Here's how the part is built. I have some questions about the finished solid (model axes, mm). A direction names the side the tool comes from. Coordinates: 2 decimals unless noted, no trailing zeros. Order: outer loops, then holes, each group sorted by start corner. A loop starts at its lowest first (then second) coordinate and runs counter-clockwise, first axis right, second up.
Autodesk Inventor part; units mm, degrees
ref_plane "YZ Plane" through (0, 0, 0) normal (1, 0, 0) x (0, 1, 0)
ref_plane "XZ Plane" through (0, 0, 0) normal (0, 1, 0) x (-1, 0, 0)
ref_plane "XY Plane" through (0, 0, 0) normal (0, 0, 1) x (1, 0, 0)
sketch "Sketch1" plane through (0, 0, 0) normal (0, 1, 0) x (-1, 0, 0)
  line L0 (-65.5034, 14.4772) -> (4.4966, 14.4772)
  line L1 (4.4966, 14.4772) -> (4.4966, -155.5228)
  line L2 (4.4966, -155.5228) -> (-65.5034, -155.5228)
  line L3 (-65.5034, -155.5228) -> (-65.5034, 14.4772)
  line L4 (4.4966, -70.5228) -> (-65.5034, -70.5228) construction
  line L5 (-30.5034, 14.4772) -> (-30.5034, -155.5228) construction
  line L6 (4.4966, -25.5228) -> (9.4966, -25.5228)
  line L7 (9.4966, -55.5228) -> (4.4966, -55.5228)
  line L8 (4.4966, -55.5228) -> (4.4966, -25.5228)
  line L9 (4.4966, -85.5228) -> (9.4966, -85.5228)
  line L10 (9.4966, -115.5228) -> (4.4966, -115.5228)
  line L11 (4.4966, -115.5228) -> (4.4966, -85.5228)
  line L12 (-5.5034, 14.4772) -> (-25.5034, 14.4772)
  line L13 (-25.5034, 14.4772) -> (-25.5034, 19.4772)
  line L14 (-25.5034, 19.4772) -> (-5.5034, 19.4772)
  line L15 (-5.5034, 19.4772) -> (-5.5034, 14.4772)
  line L16 (-55.5034, 14.4772) -> (-35.5034, 14.4772)
  line L17 (-35.5034, 14.4772) -> (-35.5034, 19.4772)
  line L18 (-35.5034, 19.4772) -> (-55.5034, 19.4772)
  line L19 (-55.5034, 19.4772) -> (-55.5034, 14.4772)
  line L20 (-65.5034, -25.5228) -> (-70.5034, -25.5228)
  line L21 (-70.5034, -25.5228) -> (-70.5034, -55.5228)
  line L22 (-70.5034, -55.5228) -> (-65.5034, -55.5228)
  line L23 (-65.5034, -85.5228) -> (-70.5034, -85.5228)
  line L24 (-70.5034, -85.5228) -> (-70.5034, -115.5228)
  line L25 (-70.5034, -115.5228) -> (-65.5034, -115.5228)
  line L26 (-25.5034, -155.5228) -> (-25.5034, -160.5228)
  line L27 (-25.5034, -160.5228) -> (-5.5034, -160.5228)
  line L28 (-5.5034, -160.5228) -> (-5.5034, -155.5228)
  line L29 (-35.5034, -155.5228) -> (-35.5034, -160.5228)
  line L30 (-35.5034, -160.5228) -> (-55.5034, -160.5228)
  line L31 (-55.5034, -160.5228) -> (-55.5034, -155.5228)
  line L32 (4.4966, 14.4772) -> (9.4966, 14.4772)
  line L33 (9.4966, -155.5228) -> (4.4966, -155.5228)
  line L34 (4.4966, -155.5228) -> (4.4966, 14.4772)
  line L35 (9.4966, 14.4772) -> (9.4966, -25.5228)
  line L36 (9.4966, -55.5228) -> (9.4966, -85.5228)
  line L37 (9.4966, -115.5228) -> (9.4966, -155.5228)
  point P0 (0, 0)
  dimension "d0" = 170
  dimension "d1" = 70
  dimension "d2" = 5
  dimension "d3" = 30
  dimension "d4" = 5
  dimension "d5" = 30
  dimension "d6" = 30
  dimension "d7" = 15
  dimension "d8" = 20
  dimension "d9" = 20
  dimension "d10" = 5
  dimension "d11" = 5
  dimension "d12" = 10
  dimension "d13" = 5
extrude "Extrusion1" add sketch "Sketch1" along normal blind 5
properties part number "LAT 4"
Q1. For faces 5 (the flat face through (-7, 2, -85.523)), 6 (the flat face through (68, 2, -85.523)), 7 (the flat face through (55.503, 2, -158)), 8 (the flat face through (5.503, 2, 17)), which set-ups out of +Z, -Z, +X, -X, +Y, -Y let a thin tool reach every point of the face, with its end or its side?
Q2. Will these pins go through, and if not, where does the flat tip stop? pin 1 (4 mm diameter, centred on x = 14.5, z = -35.5, fed in from -Y); pin 2 (2.5 mm diameter, centred on x = 0.5, y = 2, fed in from -Z); pin 3 (1.5 mm diameter, centred on y = 2.5, z = -97.5, fed in from -X); pin 4 (1.5 mm diameter, centred on y = 3.5, z = -157.5, fed in from +X).
Q3. I need wall thicknesses on L1, parallel to X at y = 3.6, z = -112; L2, parallel to X at y = 1.8, z = -11.5; L3, parallel to Z at x = 28, y = 2.15. Which ranges of each line are inside material? Lowest first, please.
Q4. If we section it at A-A on x = 0.5: Write out the boundary of the cut face in (y, z).
Q5. We'd pull the mould along X, two halves only. Please class faces 1 (the flat face through (30, 2, -155.523)), 2 (the flat face through (35.503, 2, -158)), 3 (the flat face through (70.503, 2, -40)), 4 (the flat face through (-9.497, 2, -135)): pulls with the +X half, pulls with the -X half, needs draft (parallel to the pull), parting line crosses it, or undercut.
Q6. If we section it at B-B on z = 4: Write out the boundary of the cut face in (x, y), then the cut area to 3 significant figures.
Reply:
1. face 5: -X, +Y, -Y
1. face 6: +X, +Y, -Y
1. face 7: -Z, +X, +Y, -Y
1. face 8: +Z, -X, +Y, -Y
2. pin 1: stops at y = 0
2. pin 2: stops at z = -155.52
2. pin 3: stops at x = -4.5
2. pin 4: stops at x = 55.5
3. L1: x = -4.5 to 70.5
3. L2: x = -9.5 to 65.5
3. L3: z = -155.52 to 14.48
4. outline: (0, -155.52) - (5, -155.52) - (5, 14.48) - (0, 14.48) - close
5. face 1: undercut
5. face 2: undercut
5. face 3: pulls with the +X half
5. face 4: pulls with the -X half
6. outline: (-9.5, 0) - (65.5, 0) - (65.5, 5) - (-9.5, 5) - close
6. area: 375 mm2
